Design review of the part built by this model. Coordinates are the model's own, in mm. A direction names the side the tool comes from. Coordinates: 2 decimals unless noted, no trailing zeros. Write each loop counter-clockwise with the first axis right and the second up, starting at its lowest first coordinate (ties: lowest second). Pieces come first, ordered by that corner, then holes. Notation, with made-up numbers: (40.5, -27.5) -> (55.5, -27.5) arc R9 cw to (55.5, -17.5) -> close; hole circle Ø2 at (69.25, 79.5). An arc over 180 degrees is marked (long way). Return JSON: item names as keys, results as strings. Group by question number.
from build123d import *

# Parameters (mm, degrees)
SKETCH1_R             = 3.4
BOSS_EXTRUDE1_DEPTH   = 30
BOSS_EXTRUDE1_2_DEPTH = 30
BOSS_EXTRUDE1_3_DEPTH = 30
BOSS_EXTRUDE1_4_DEPTH = 30
BOSS_EXTRUDE2_DEPTH   = 5
CUT_EXTRUDE1_REACH    = 69.93
FILLET1_R             = 3


with BuildPart() as part:
    # Sketch1 → Boss-Extrude1 (new body)
    with BuildSketch(Plane.XY):
        with Locations((29, -40)):
            Circle(SKETCH1_R)
    extrude(amount=BOSS_EXTRUDE1_DEPTH)



with BuildPart() as body_2:
    # Sketch1 → Boss-Extrude1 2 (new body)
    with BuildSketch(Plane.XY):
        with Locations((-29, -40)):
            Circle(SKETCH1_R)
    extrude(amount=BOSS_EXTRUDE1_2_DEPTH)


with BuildPart() as body_3:
    # Sketch1 → Boss-Extrude1 3 (new body)
    with BuildSketch(Plane.XY):
        with Locations((-29, 9)):
            Circle(SKETCH1_R)
    extrude(amount=BOSS_EXTRUDE1_3_DEPTH)


with BuildPart() as body_4:
    # Sketch1 → Boss-Extrude1 4 (new body)
    with BuildSketch(Plane.XY):
        with Locations((29, 9)):
            Circle(SKETCH1_R)
    extrude(amount=BOSS_EXTRUDE1_4_DEPTH)


with BuildPart() as part_1:
    add(part.part)

    add(body_2.part)  # Boss-Extrude2 merges body 2

    add(body_3.part)  # Boss-Extrude2 merges body 3

    add(body_4.part)  # Boss-Extrude2 merges body 4
    # Sketch2 → Boss-Extrude2 (add)
    with BuildSketch(Plane.XY.offset(30)):
        with BuildLine():
            Line((-24.85, -50), (24.85, -50))
            ThreePointArc((24.85, -50), (31.921067812, -47.071067812), (34.85, -40))
            Line((34.85, -40), (34.85, 20))
            Line((34.85, 20), (-34.85, 20))
            Line((-34.85, 20), (-34.85, -40))
            ThreePointArc((-34.85, -40), (-31.921067812, -47.071067812), (-24.85, -50))
        make_face()
    extrude(amount=BOSS_EXTRUDE2_DEPTH)

    # Sketch3 → Cut-Extrude1 (cut, up to next)
    with BuildSketch(Plane(origin=(0, 0, 30), x_dir=(-1, 0, 0), z_dir=(0, 0, -1)), mode=Mode.PRIVATE) as cut_extrude1_sk1:
        Polygon((-5.268445512, -15.5), (-31.194195607, 6.402788873), (-31.194195607, -37.402788873), align=None)
    cut_extrude1_tool1 = extrude(cut_extrude1_sk1.sketch, amount=-CUT_EXTRUDE1_REACH, mode=Mode.PRIVATE) & part_1.part
    # Sketch3 → Cut-Extrude1 (cut, up to next)
    with BuildSketch(Plane(origin=(0, 0, 30), x_dir=(-1, 0, 0), z_dir=(0, 0, -1)), mode=Mode.PRIVATE) as cut_extrude1_sk2:
        Polygon((26.805804393, 11.597211127), (-26.805804393, 11.597211127), (0, -11.049071895), align=None)
    cut_extrude1_tool2 = extrude(cut_extrude1_sk2.sketch, amount=-CUT_EXTRUDE1_REACH, mode=Mode.PRIVATE) & part_1.part
    # Sketch3 → Cut-Extrude1 (cut, up to next)
    with BuildSketch(Plane(origin=(0, 0, 30), x_dir=(-1, 0, 0), z_dir=(0, 0, -1)), mode=Mode.PRIVATE) as cut_extrude1_sk3:
        Polygon((31.194195607, 6.402788873), (5.268445512, -15.5), (31.194195607, -37.402788873), align=None)
    cut_extrude1_tool3 = extrude(cut_extrude1_sk3.sketch, amount=-CUT_EXTRUDE1_REACH, mode=Mode.PRIVATE) & part_1.part
    # Sketch3 → Cut-Extrude1 (cut, up to next)
    with BuildSketch(Plane(origin=(0, 0, 30), x_dir=(-1, 0, 0), z_dir=(0, 0, -1)), mode=Mode.PRIVATE) as cut_extrude1_sk4:
        Polygon((26.805804393, -42.597211127), (0, -19.950928105), (-26.805804393, -42.597211127), align=None)
    cut_extrude1_tool4 = extrude(cut_extrude1_sk4.sketch, amount=-CUT_EXTRUDE1_REACH, mode=Mode.PRIVATE) & part_1.part
    add(cut_extrude1_tool1.solids().sort_by_distance((22.552279, -15.5, 30))[0], mode=Mode.SUBTRACT)
    add(cut_extrude1_tool2.solids().sort_by_distance((0, 4.04845, 30))[0], mode=Mode.SUBTRACT)
    add(cut_extrude1_tool3.solids().sort_by_distance((-22.552279, -15.5, 30))[0], mode=Mode.SUBTRACT)
    add(cut_extrude1_tool4.solids().sort_by_distance((0, -35.04845, 30))[0], mode=Mode.SUBTRACT)

    # Fillet1
    # the kernel refuses this fillet: 3 mm, written as the material it adds along each edge
    with BuildSketch(Plane(origin=(-31.194195607, 6.402788873, 30), x_dir=(0, -1, 0), z_dir=(0, 0, 1)), Plane(origin=(31.194195607, -37.402788873, 30), x_dir=(0, 1, 0), z_dir=(0, 0, 1))) as fillet1_piece_1:
        with BuildLine():
            CenterArc((FILLET1_R * 2.15392408777, FILLET1_R), FILLET1_R, 139.807953963, 130.192046037)
            Line((FILLET1_R * 1.39003846223, FILLET1_R * 1.64535164917), (0, 0))
            Line((0, 0), (FILLET1_R * 2.15392408777, 0))
        make_face()
    extrude(amount=5)
    with BuildSketch(Plane(origin=(-31.194195607, -37.402788873, 30), x_dir=(0, 1, 0), z_dir=(0, 0, 1)), Plane(origin=(31.194195607, 6.402788873, 30), x_dir=(0, -1, 0), z_dir=(0, 0, 1))) as fillet1_piece_2:
        with BuildLine():
            CenterArc((FILLET1_R * 2.15392408777, -FILLET1_R), FILLET1_R, 90, 130.192046037)
            Line((FILLET1_R * 1.39003846223, -FILLET1_R * 1.64535164917), (0, 0))
            Line((0, 0), (FILLET1_R * 2.15392408777, 0))
        make_face()
    extrude(amount=5)
    with BuildSketch(Plane(origin=(-5.268445512, -15.5, 30), x_dir=(-0.7638856255460464, -0.6453516491682078, 0), z_dir=(0, 0, 1))) as fillet1_piece_3:
        with BuildLine():
            CenterArc((FILLET1_R * 1.18367346939, -FILLET1_R), FILLET1_R, 90, 99.615907926)
            Line((FILLET1_R * 0.197723772944, -FILLET1_R * 1.16704249783), (0, 0))
            Line((0, 0), (FILLET1_R * 1.18367346939, 0))
        make_face()
    extrude(amount=5)
    with BuildSketch(Plane(origin=(-26.805804393, 11.597211127, 30), x_dir=(1, 0, 0), z_dir=(0, 0, 1)), Plane(origin=(26.805804393, -42.597211127, 30), x_dir=(-1, 0, 0), z_dir=(0, 0, 1))) as fillet1_piece_4:
        with BuildLine():
            CenterArc((FILLET1_R * 2.73321626716, -FILLET1_R), FILLET1_R, 90, 139.807953963)
            Line((FILLET1_R * 2.08786461799, -FILLET1_R * 1.76388562555), (0, 0))
            Line((0, 0), (FILLET1_R * 2.73321626716, 0))
        make_face()
    extrude(amount=5)
    with BuildSketch(Plane(origin=(0, -11.049071895, 30), x_dir=(0.7638856255460464, 0.6453516491682076, 0), z_dir=(0, 0, 1))) as fillet1_piece_5:
        with BuildLine():
            CenterArc((FILLET1_R * 0.844827586207, FILLET1_R), FILLET1_R, 189.615907926, 80.384092074)
            Line((-FILLET1_R * 0.141122110237, FILLET1_R * 0.832957502168), (0, 0))
            Line((0, 0), (FILLET1_R * 0.844827586207, 0))
        make_face()
    extrude(amount=5)
    with BuildSketch(Plane(origin=(26.805804393, 11.597211127, 30), x_dir=(-1, 0, 0), z_dir=(0, 0, 1)), Plane(origin=(-26.805804393, -42.597211127, 30), x_dir=(1, 0, 0), z_dir=(0, 0, 1))) as fillet1_piece_6:
        with BuildLine():
            CenterArc((FILLET1_R * 2.73321626716, FILLET1_R), FILLET1_R, 130.192046037, 139.807953963)
            Line((FILLET1_R * 2.08786461799, FILLET1_R * 1.76388562555), (0, 0))
            Line((0, 0), (FILLET1_R * 2.73321626716, 0))
        make_face()
    extrude(amount=5)
    with BuildSketch(Plane(origin=(0, -19.950928105, 30), x_dir=(0.7638856255460446, -0.6453516491682099, 0), z_dir=(0, 0, 1))) as fillet1_piece_7:
        with BuildLine():
            CenterArc((FILLET1_R * 0.844827586207, -FILLET1_R), FILLET1_R, 90, 80.384092074)
            Line((-FILLET1_R * 0.141122110237, -FILLET1_R * 0.832957502168), (0, 0))
            Line((0, 0), (FILLET1_R * 0.844827586207, 0))
        make_face()
    extrude(amount=5)
    with BuildSketch(Plane(origin=(5.268445512, -15.5, 30), x_dir=(0.7638856255460458, -0.6453516491682085, 0), z_dir=(0, 0, 1))) as fillet1_piece_8:
        with BuildLine():
            CenterArc((FILLET1_R * 1.18367346939, FILLET1_R), FILLET1_R, 170.384092074, 99.615907926)
            Line((FILLET1_R * 0.197723772944, FILLET1_R * 1.16704249783), (0, 0))
            Line((0, 0), (FILLET1_R * 1.18367346939, 0))
        make_face()
    extrude(amount=5)


solid = part_1.part
Q1. We need section B-B on z = 15. Write out the cut boundary in (x, y).
Q2. For faces 1 (the flat face through (-2, -15, 35)), 2 (the flat face through (17.25, -25.62, 32.47)), 3 (the cylindrical face through (-25.86, 7.7, 14.79)), list the 3-axis set-ups (+Z, -Z, +X, -X, +Y, -Y) from which the entire face can be reached by the end or side of a thin tool; tool diameter is ignored.
Q3. The part is to be moulded in two halves that separate along X. For faces 4 (the flat face through (-34.85, -10, 32)), 5 (the flat face through (0, -50, 32)), 6 (the cylindrical face through (6.917, -15.463, 32.465)), say which applies: +X half, -X half, draft (parallel to the pull), parting line (faces both ways), or undercut.
Q4. Wall thickness on L1, parallel to Y at x = 0, z = 33.5; L2, parallel to Z at x = 30, y = -34; L3, parallel to Y at x = 29, z = 11: over which ranges is each line inside the solid? List them lowest first.
Q5. We need section A-A on y = -3. Write out the cut boundary in (x, z).
Q6. For P1, Ø1, axis at y = 11.5, z = 21.5, coming from the +X side; P2, Ø1, axis at x = 25, y = -35, coming from the -Z side; P3, Ø5, axis at x = 25, z = 20, coming from the -Y side; P4, Ø5, axis at x = 22.5, y = -26, coming from the -Z side, all flat-tipped, find the tip position at first contact; note any pin that passes through.
Q7. We need section C-C on x = 29. Write out the cut boundary in (y, z).
Q8. We need section D-D on y = 9. Write out the cut boundary in (x, z).
Findings below:
{
 "1": {"outline": "circle Ø6.8 at (-29, -40); circle Ø6.8 at (-29, 9); circle Ø6.8 at (29, -40); circle Ø6.8 at (29, 9)"},
 "2": {"face 1": "+Z, +X, -X, +Y, -Y", "face 2": "+Z, -Z", "face 3": "-Z"},
 "3": {"face 4": "-X half", "face 5": "draft", "face 6": "undercut"},
 "4": {"L1": "y = -50 to -42.6, -20.88 to -10.12, 11.6 to 20", "L2": "z = 30 to 35", "L3": "y = -43.4 to -36.6, 5.6 to 12.4"},
 "5": {"outline": "(-34.85, 30) -> (-31.19, 30) -> (-31.19, 35) -> (-34.85, 35) -> close; (-20.06, 30) -> (-9.53, 30) -> (-9.53, 35) -> (-20.06, 35) -> close; (9.53, 30) -> (20.06, 30) -> (20.06, 35) -> (9.53, 35) -> close; (31.19, 30) -> (34.85, 30) -> (34.85, 35) -> (31.19, 35) -> close"},
 "6": {"P1": "stops at x = 31.75", "P2": "stops at z = 30", "P3": "stops at y = -43.05", "P4": "passes through"},
 "7": {"outline": "(-49.1, 30) -> (-43.4, 30) -> (-43.4, 0) -> (-36.6, 0) -> (-36.6, 30) -> (-33.83, 30) -> (-33.83, 35) -> (-49.1, 35) -> close; (2.83, 30) -> (5.6, 30) -> (5.6, 0) -> (12.4, 0) -> (12.4, 30) -> (20, 30) -> (20, 35) -> (2.83, 35) -> close"},
 "8": {"outline": "(-34.85, 30) -> (-32.4, 30) -> (-32.4, 0) -> (-25.6, 0) -> (-25.6, 30) -> (-21.58, 30) -> (-21.58, 35) -> (-34.85, 35) -> close; (21.58, 30) -> (25.6, 30) -> (25.6, 0) -> (32.4, 0) -> (32.4, 30) -> (34.85, 30) -> (34.85, 35) -> (21.58, 35) -> close"}
}
